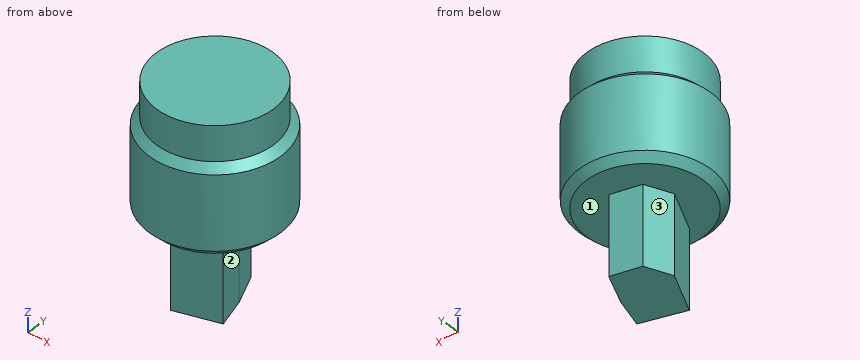
from build123d import *

# Parameters (mm, degrees)
F0_R     = 45.2513140414
F1_DEPTH = 36.2754836679
F3_DEPTH = 38.2841601968
F5_DEPTH = 24.6460158378
F6_SIZE  = 5.08
F7_DEPTH = 23.8733459264
F8_DEPTH = 16.1826983094


with BuildPart() as f1:
    # F0 (on Top) → F1 (new body)
    with BuildSketch(Plane.XY):
        Circle(F0_R)
    extrude(amount=F1_DEPTH)

    # F2 (on face) → F3 (join)
    with BuildSketch(Plane(origin=(0, 0, 0), x_dir=(1, 0, 0), z_dir=(0, 0, -1))):
        Polygon((-12.9493158311, -17.3341035843), (6.9733597338, -21.838657558), (16.743408516, 0), (22.6436909288, 20.306520164), (-6.7410551447, 28.8445807998), (-20.420435816, 0), align=None)
    extrude(amount=F3_DEPTH)

    # F5 (add): a face of the model
    f5_faces = [f1.faces().sort_by_distance(p)[0] for p in [
        (0, 0, 36.2754836679),
    ]]
    extrude(f5_faces, amount=F5_DEPTH)

    # F6
    f6_edges = [f1.edges().sort_by_distance(p)[0] for p in [
        (-45.251314, 0, 60.9215),
        (-45.251314, 0, 0),
        (45.251314, 0, 30.46075),
    ]]
    chamfer(f6_edges, length=F6_SIZE)

    # F7 (add): a face of the model
    f7_faces = [f1.faces().sort_by_distance(p)[0] for p in [
        (0, 0, 60.9214995056),
    ]]
    extrude(f7_faces, amount=F7_DEPTH)

    # F4 (on face) → F8 (join)
    with BuildSketch(Plane(origin=(0, 0, -38.2841601968), x_dir=(1, 0, 0), z_dir=(0, 0, -1))):
        Polygon((22.6436909288, 20.306520164), (-6.7410551447, 28.8445807998), (-20.420435816, 0), (-12.9493158311, -17.3341035843), (6.9733597338, -21.838657558), (16.743408516, 0), align=None)
    extrude(amount=F8_DEPTH)


solid = f1.part
Geometry: final body of the model. Coordinates: model frame, mm. Face numbers are marked on the shaded views. A direction names the side the tool comes from. Round coordinates to 2 decimals unless told otherwise and drop trailing zeros. Loops run counter-clockwise (first coordinate to the right, second up) from the corner with the lowest first, then second, coordinate; pieces in that order, holes last. Notation, with made-up numbers: M -25,72.25 L -5,72.25 A19 cw -5,81.25 Z; hole C 49.5,68 d9. An arc over 180 degrees is marked long. One line per question, with ' | ' between items.
(1) Access query for the marked faces 1, 2 and 3. Directions: +Z, -Z, +X, -X, +Y, -Y. A direction counts if a zero-diameter tool reaches every point of the face in a straight line with its end or side. Return the directions, or none.
Check result:
face 1: -Z | face 2: -Z, +X, +Y | face 3: -Z, -X, +Y
(2) Cut plane B-B on z = 11. Return the cut outline in (x, y), plus the area to 3 significant figures.
Check result:
outline: C 0,0 d90.5 | area: 6,430 mm2
(3) Contact query for flat-ended pins moving along their axis: P1, Ø10, axis at x = -33, z = 34, coming from the -Y side; P2, Ø3, axis at x = -28, y = -22, coming from the -Z side; P3, Ø2, axis at y = 30.5, z = 9.5, coming from the -X side. Output: stop coordinate, or through.
Check result:
P1: stops at y = -35.55 | P2: stops at z = 0 | P3: stops at x = -34.31
(4) Cut plane A-A on x = 0. Return the cut outline in (y, z), plus the area to 3 significant figures.
Check result:
outline: M -45.25,5.08 L -40.17,0 L -26.89,0 L -26.89,-54.47 L 20.26,-54.47 L 20.26,0 L 40.17,0 L 45.25,5.08 L 45.25,55.84 L 40.17,60.92 L 40.17,84.79 L -40.17,84.79 L -40.17,60.92 L -45.25,55.84 Z | area: 9,950 mm2
(5) Material intervals for line 1 along Z through (x, y) = (-14.5, 33.5); line 2 along X through (y, z) = (6, 53.5); line 3 along Y through (x, z) = (-32.5, 64), sorted ascending. Write a range as from..to.
Check result:
line 1: z = 0..84.79 | line 2: x = -44.85..44.85 | line 3: y = -23.61..23.61
